Could you check a few things on this model? Use its own coordinates, in mm. Face numbers are marked on the shaded views. A direction names the side the tool comes from. Coordinates: 2 decimals unless noted, no trailing zeros.
from build123d import *

# Parameters (mm, degrees)
PAD_DEPTH       = 5
PAD001_DEPTH    = 120
POCKET_DEPTH    = 125
POCKET001_DEPTH = 5
SKETCH005_W     = 65
SKETCH005_H     = 14.081008
POCKET002_DEPTH = 50
SKETCH006_W     = 50
SKETCH006_H     = 12.788605
POCKET003_DEPTH = 41
PAD003_DEPTH    = 84
PAD004_DEPTH    = 20


with BuildPart() as part:
    # Sketch → Pad (new body)
    with BuildSketch(Plane.XY):
        with BuildLine():
            Line((-37.700377, -64.976087), (37.645855, -64.976087))
            ThreePointArc((37.645855, -64.976087), (48.132338, -60.632444), (52.475981, -50.145961))
            Line((52.475981, -50.145961), (52.475981, 50.144628))
            ThreePointArc((52.475981, 50.144628), (48.132338, 60.63111), (37.645855, 64.974754))
            Line((37.645855, 64.974754), (-37.689561, 64.974754))
            ThreePointArc((-37.689561, 64.974754), (-48.173873, 60.63328), (-52.519686, 50.150766))
            Line((-52.519686, 50.150766), (-61.964051, 50.150766))
            ThreePointArc((-61.964051, 50.150766), (-63.064051, 49.695131), (-63.519686, 48.595131))
            Line((-63.519686, 48.595131), (-63.519686, -49.156657))
            ThreePointArc((-63.519686, -49.156657), (-63.064051, -50.256657), (-61.964051, -50.712292))
            Line((-52.519686, -50.712292), (-61.964051, -50.712292))
            ThreePointArc((-52.519686, -50.712292), (-47.984683, -60.830796), (-37.700377, -64.976087))
        make_face()
    extrude(amount=PAD_DEPTH)

    # Sketch001 (on Face14 of Pad) → Pad001 (join)
    with BuildSketch(Plane.XY.offset(5)):
        with BuildLine():
            Line((-37.672841, -65), (37.643326, -65))
            ThreePointArc((37.643326, -65), (48.148581, -60.648581), (52.5, -50.143326))
            Line((52.5, -50.143326), (52.5, 50.143326))
            ThreePointArc((52.5, 50.143326), (48.148581, 60.648581), (37.643326, 65))
            Line((37.643326, 65), (-37.662754, 65))
            ThreePointArc((-37.662754, 65), (-48.168272, 60.648318), (-52.519428, 50.142583))
            Line((-52.519428, 50.142583), (-61.967391, 50.142583))
            ThreePointArc((-61.967391, 50.142583), (-63.064847, 49.688002), (-63.519428, 48.590546))
            Line((-63.519428, 48.590546), (-63.519428, -49.13867))
            ThreePointArc((-63.519428, -49.13867), (-63.064847, -50.236126), (-61.967391, -50.690707))
            Line((-52.519428, -50.690707), (-61.967391, -50.690707))
            ThreePointArc((-52.519428, -50.690707), (-47.982752, -60.840359), (-37.672841, -65))
        make_face()
        with BuildLine():
            Line((-35.860247, -62.5), (35.860247, -62.5))
            ThreePointArc((35.860247, -62.5), (45.858562, -58.358562), (50, -48.360247))
            Line((50, -48.360247), (50, 48.360247))
            ThreePointArc((50, 48.360247), (45.858562, 58.358562), (35.860247, 62.5))
            Line((35.860247, 62.5), (-35.860247, 62.5))
            ThreePointArc((-35.860247, 62.5), (-45.858562, 58.358562), (-50, 48.360247))
            Line((-50, 48.360247), (-50, -48.360247))
            ThreePointArc((-50, -48.360247), (-45.858562, -58.358562), (-35.860247, -62.5))
        make_face(mode=Mode.SUBTRACT)
    extrude(amount=PAD001_DEPTH)

    # Sketch002 (on Face4 of Pad001) → Pocket (cut)
    with BuildSketch(Plane(origin=(0, 0, 0), x_dir=(1, 0, 0), z_dir=(0, 0, -1))):
        with BuildLine():
            Line((-63.519686, 40), (-63.519686, -40))
            Line((-63.519686, -40), (-60.519686, -40))
            Line((-60.519686, -40), (-60.519686, -44.345519))
            ThreePointArc((-60.519686, -44.345519), (-60.327906, -44.808517), (-59.864908, -45.000297))
            Line((-59.864908, -45.000297), (-56.174464, -45.000297))
            ThreePointArc((-56.174464, -45.000297), (-55.711466, -44.808517), (-55.519686, -44.345519))
            Line((-55.519686, -44.345519), (-55.519686, -40))
            Line((-55.519686, -40), (-48.593648, -40))
            Line((-48.593648, -40), (-48.593648, 40.000547))
            Line((-55.593648, 40.000547), (-48.593648, 40.000547))
            Line((-55.593648, 44.345222), (-55.593648, 40.000547))
            ThreePointArc((-55.593648, 44.345222), (-55.785428, 44.80822), (-56.248426, 45))
            Line((-59.864908, 45), (-56.248426, 45))
            ThreePointArc((-59.864908, 45), (-60.327906, 44.80822), (-60.519686, 44.345222))
            Line((-60.519686, 40), (-60.519686, 44.345222))
            Line((-63.519686, 40), (-60.519686, 40))
        make_face()
    extrude(amount=-POCKET_DEPTH, mode=Mode.SUBTRACT)

    # Sketch003 (on Face4 of Pocket) → Pocket001 (cut)
    with BuildSketch(Plane(origin=(0, 0, 0), x_dir=(1, 0, 0), z_dir=(0, 0, -1))):
        with BuildLine():
            ThreePointArc((0, -30.099214), (30.047141, -0.048909), (0, 30.001395))
            Line((0, 30.001395), (-50, 30.001395))
            Line((-50, -30.099214), (-50, 30.001395))
            Line((0, -30.099214), (-50, -30.099214))
        make_face()
    extrude(amount=-POCKET001_DEPTH, mode=Mode.SUBTRACT)

    # Sketch005 (on Face46 of Pocket001) → Pocket002 (cut)
    with BuildSketch(Plane.XY.offset(125)):
        with Locations((0, 65.410759)):
            Rectangle(SKETCH005_W, SKETCH005_H)
    extrude(amount=-POCKET002_DEPTH, mode=Mode.SUBTRACT)

    # Sketch006 (on Face46 of Pocket002) → Pocket003 (cut)
    with BuildSketch(Plane.XY.offset(125)):
        with Locations((0, -63.418121)):
            Rectangle(SKETCH006_W, SKETCH006_H)
    extrude(amount=-POCKET003_DEPTH, mode=Mode.SUBTRACT)

    # Sketch007 (on Face4 of Pocket003) → Pad003 (join)
    with BuildSketch(Plane(origin=(0, 0, 0), x_dir=(1, 0, 0), z_dir=(0, 0, -1))):
        Polygon((-0.027261, 64.976087), (-25.027261, 64.976087), (-25.027261, 74.976087), (24.972739, 74.976087), (24.972739, 64.976087), align=None)
    extrude(amount=-PAD003_DEPTH)

    # Sketch009 (on Face73 of Pad003) → Pad004 (join)
    with BuildSketch(Plane.XY.offset(84)):
        Polygon((-25, -62.5), (-25, -74.976087), (24.972739, -74.976087), (24.972739, -62.5), (21, -62.5), (21, -72.5), (-20, -72.5), (-20, -62.5), align=None)
    extrude(amount=PAD004_DEPTH)


solid = part.part
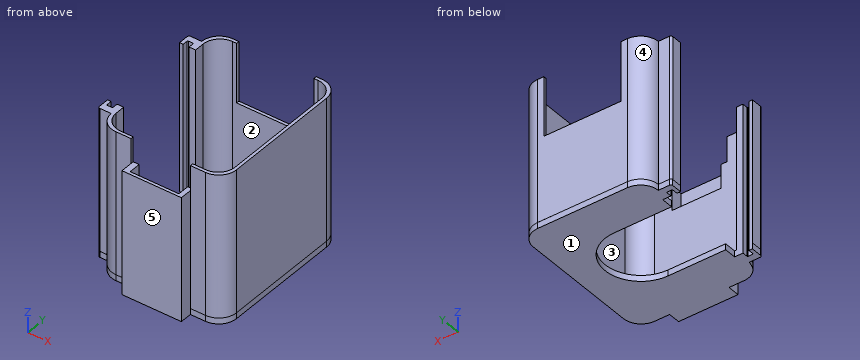
1) Will these pins go through, and if not, where does the flat tip stop? pin 1 (4 mm diameter, centred on y = -6, z = 2.5, fed in from +X); pin 2 (1.5 mm diameter, centred on x = -56, z = 3, fed in from +Y); pin 3 (1.5 mm diameter, centred on x = -30.5, z = 3, fed in from -Y).
2) For the marked faces 1 and 2, which set-ups out of +Z, -Z, +X, -X, +Y, -Y let a thin tool reach every point of the face, with its end or its side?
3) Imagine slicing it at B-B on z = 98.5. State how many separate pieces and enclosed holes the cut face has, plus the area to 3 significant figures.
4) If I drill on L1, parallel to X at y = -44, z = 78; L2, parallel to Y at x = 6, z = 20; L3, parallel to Y at x = 27, z = 52, over which ranges is the centre line in solid material (lowest first)?
5) We'd pull the mould along Y, two halves only. Please class the marked faces 3, 4 and 5: released by +Y, released by -Y, zero draft, split by the parting line, or undercut.
Solved:
1. pin 1: stops at x = 52.48
1. pin 2: stops at y = 50.15
1. pin 3: stops at y = -64.98
2. face 1: -Z, +X, -X, +Y, -Y
2. face 2: +Z
3. separate pieces: 3
3. enclosed holes: 0
3. area: 1,040 mm2
4. L1: x = -63.52 to -60.52, -55.59 to -50, 50 to 52.5
4. L2: y = -74.98 to -62.5, 62.5 to 65
4. L3: y = -65 to -62.5, 62.5 to 65
5. face 3: undercut
5. face 4: released by +Y
5. face 5: released by -Y
